Here's how the part is built. I have some questions about the finished solid (model axes, mm). A direction names the side the tool comes from. Round coordinates to 2 decimals unless told otherwise and drop trailing zeros. Order: outer loops, then holes, each group sorted by start corner. A loop starts at its lowest first (then second) coordinate and runs counter-clockwise, first axis right, second up.
```python
from build123d import *

# Parameters (mm, degrees)
F0_W      = 65
F0_H      = 20
F1_DEPTH  = 7
F2_D      = 5
F3_R      = 3.5
F4_DEPTH  = 25
F6_D      = 2.4
F6_DEPTH  = 11.8
F6_TIP    = 0.7210327428
F8_R      = 5.5
F9_DEPTH  = 25
F10_R     = 3.5
F11_DEPTH = 5


# Not quite as in the source:
# - a pattern or mirror of a feature is missing from the dataset's text; its kind, count and spacing are read off the source's solid


with BuildPart() as f1:
    # F0 (on Top) → F1 (new body)
    with BuildSketch(Plane.XY):
        with BuildLine():
            ThreePointArc((9, 27), (8.4142135624, 28.4142135624), (7, 29))
            Line((7, 29), (-72, 29))
            ThreePointArc((-72, 29), (-73.4142135624, 28.4142135624), (-74, 27))
            Line((-74, 27), (-74, -7))
            ThreePointArc((-74, -7), (-73.4142135624, -8.4142135624), (-72, -9))
            Line((-72, -9), (7, -9))
            ThreePointArc((7, -9), (8.4142135624, -8.4142135624), (9, -7))
            Line((9, -7), (9, 27))
        make_face()
        with Locations((-32.5, 10)):
            Rectangle(F0_W, F0_H, mode=Mode.SUBTRACT)
        with Locations((-32.5, 10)):
            Rectangle(F0_W, F0_H)
    extrude(amount=F1_DEPTH)

    # F2 (through all)
    with Locations(Plane(origin=(0, 0, 0), x_dir=(1, 0, 0), z_dir=(0, 0, -1))):
        with Locations((-65, -20), (-65, 0), (0, 0), (0, -20)):
            Hole(F2_D / 2)

    # F3 (on face) → F4 (cut)
    with BuildSketch(Plane.XY.offset(7)):
        with Locations((-62.5, 10)):
            Circle(F3_R)
        with Locations((-2.5, 10)):
            Circle(F3_R)
    extrude(amount=-F4_DEPTH, mode=Mode.SUBTRACT)

    # F6
    with Locations(Plane.YZ.offset(9)):
        with Locations((10, 3.5)):
            f6 = Hole(F6_D / 2, depth=F6_DEPTH)
            with Locations((0, 0, -(F6_DEPTH + F6_TIP / 2))):  # 118° drill point
                Cone(0, F6_D / 2, F6_TIP, mode=Mode.SUBTRACT)

    # F6_copies: F6 across plane
    add(f6.mirror(Plane(origin=(-32.500003, -1e-06, 0), x_dir=(0, 0, -1), z_dir=(-1, 0, 0))), mode=Mode.SUBTRACT)

    # F8 (on face) → F9 (cut)
    with BuildSketch(Plane.XY.offset(7)):
        with Locations((-32.5, 10)):
            Circle(F8_R)
    extrude(amount=-F9_DEPTH, mode=Mode.SUBTRACT)

    # F10 (on face) → F11 (cut)
    with BuildSketch(Plane.XY):
        Circle(F10_R)
        with Locations((-65, 0)):
            Circle(F10_R)
        with Locations((0, 20)):
            Circle(F10_R)
        with Locations((-65, 20)):
            Circle(F10_R)
    extrude(amount=F11_DEPTH, mode=Mode.SUBTRACT)


solid = f1.part
```
1) If we section it at A-A (y = 10): Write out the boundary of the cut face in (x, z), plus the area to 3 significant figures.
2) I need wall thicknesses on line 1 (X direction, y = 20, z = 6.55); line 2 (Y direction, x = -3, z = 4); line 3 (Y direction, x = 2, z = 3.75). Which ranges of each line are inside material? Lowest first, please.
3) We'd pull the mould along X, two halves only. Please class faces 4 (the cylindrical face through (-73.4, 28.43, 3.45)), 5 (the cylindrical face through (-59.267, 8.659, 3.549)), 6 (the flat face through (9, 10, 5)): +X half, -X half, draft (parallel to the pull), parting line (faces both ways), or undercut.
4) I'm going to push a flat-ended pin straight in: pin 1 (6.5 mm diameter, centred on x = 0, y = 20, fed in from -Z). Where does the tip first touch, or does it pass through?
5) For faces 1 (the flat face through (-33, -9, 3)), 2 (the cylindrical face through (-68.497, 0.154, 2.465)), 3 (the cylindrical face through (4.84, 8.89, 3.04)), which set-ups out of +Z, -Z, +X, -X, +Y, -Y let a thin tool reach every point of the face, with its end or its side?
6) If we section it at B-B (z = 3.5): Write out the boundary of the cut face in (x, y).
7) If we section it at D-D (x = -32.5): Write out the boundary of the cut face in (y, z), plus the area to 3 significant figures.
8) If we section it at C-C (y = 0): Write out the boundary of the cut face in (x, z), plus the area to 3 significant figures.
Solutions:
1. outline: (-74, 0) - (-66, 0) - (-66, 2.3) - (-74, 2.3) - close; (-74, 4.7) - (-66, 4.7) - (-66, 7) - (-74, 7) - close; (-59, 0) - (-38, 0) - (-38, 7) - (-59, 7) - close; (-27, 0) - (-6, 0) - (-6, 7) - (-27, 7) - close; (1, 0) - (9, 0) - (9, 2.3) - (1, 2.3) - close; (1, 4.7) - (9, 4.7) - (9, 7) - (1, 7) - close
1. area: 368 mm2
2. line 1: x = -74 to -67.5, -62.5 to -2.5, 2.5 to 9
2. line 2: y = -9 to -1.8, 1.8 to 6.54, 13.46 to 18.2, 21.8 to 29
2. line 3: y = -9 to -2.87, 2.87 to 8.83, 11.17 to 17.13, 22.87 to 29
3. face 4: -X half
3. face 5: undercut
3. face 6: +X half
4. pin 1: stops at z = 5
5. face 1: +Z, -Z, +X, -X, -Y
5. face 2: -Z
5. face 3: +X
6. outline: (-74, -7) arc R2 ccw to (-72, -9) - (7, -9) arc R2 ccw to (9, -7) - (9, 8.8) - (0.79, 8.8) arc R3.5 cw (long way) to (0.79, 11.2) - (9, 11.2) - (9, 27) arc R2 ccw to (7, 29) - (-72, 29) arc R2 ccw to (-74, 27) - (-74, 11.2) - (-65.79, 11.2) arc R3.5 cw (long way) to (-65.79, 8.8) - (-74, 8.8) - close; hole circle Ø7 at (-65, 0); hole circle Ø7 at (-65, 20); hole circle Ø11 at (-32.5, 10); hole circle Ø7 at (0, 0); hole circle Ø7 at (0, 20)
7. outline: (-9, 0) - (4.5, 0) - (4.5, 7) - (-9, 7) - close; (15.5, 0) - (29, 0) - (29, 7) - (15.5, 7) - close
7. area: 189 mm2
8. outline: (-74, 0) - (-68.5, 0) - (-68.5, 5) - (-67.5, 5) - (-67.5, 7) - (-74, 7) - close; (-62.5, 5) - (-61.5, 5) - (-61.5, 0) - (-3.5, 0) - (-3.5, 5) - (-2.5, 5) - (-2.5, 7) - (-62.5, 7) - close; (2.5, 5) - (3.5, 5) - (3.5, 0) - (9, 0) - (9, 7) - (2.5, 7) - close
8. area: 491 mm2
